Geometry check sheet. Reference: the model listing, model coordinates, mm. Face numbers are marked on the shaded views. A direction names the side the tool comes from. Round coordinates to 2 decimals unless told otherwise and drop trailing zeros. Order: outer loops, then holes, each group sorted by start corner. A loop starts at its lowest first (then second) coordinate and runs counter-clockwise, first axis right, second up. Notation, with made-up numbers: (14.25, -14.75) - (50.25, -14.75) arc R19 ccw to (50.25, -5.75) - close; hole circle Ø4 at (41, 57). An arc over 180 degrees is marked (long way). Use a Markdown table: item, result. Add a question column.
(1) Gauge pin test, flat ends, axial feed: P1, Ø1.5, axis at x = 16.5, y = 3.5, coming from the +Z side; P2, Ø1, axis at y = 3, z = 8, coming from the -X side; P3, Ø1, axis at x = 11.5, z = 8, coming from the -Y side; P4, Ø2.5, axis at x = 15.75, y = 3, coming from the -Z side. Record the tip position at first contact, or that the pin passes through.
(2) Mould release check, pull along Y, two halves, no side actions. Record for the marked faces 3, 4 and 5: released by +Y, released by -Y, zero draft, split by the parting line, or undercut.
(3) Section check C-C on z = 1.75. Give the number of separate pieces and of enclosed holes in the cut face, then the cut area to 3 significant figures.
(4) Thickness scan on line 1 along Y through (x, z) = (9.5, 4); line 2 along Z through (x, y) = (15.5, 1.5); line 3 along Y through (x, z) = (2.5, 4.75). Record the ranges inside material, lowest first. Write a range as [from, to].
(5) Access from +Z, -Z, +X, -X, +Y, -Y to the whole of each face (thin tool, end or side, straight path). Record for the marked faces 1 and 2.
(6) Section check B-B on x = 3.25. Record the boundary of the cut face in (y, z).
(7) Section check A-A on z = 7.5. Record the boundary of the cut face in (x, y).
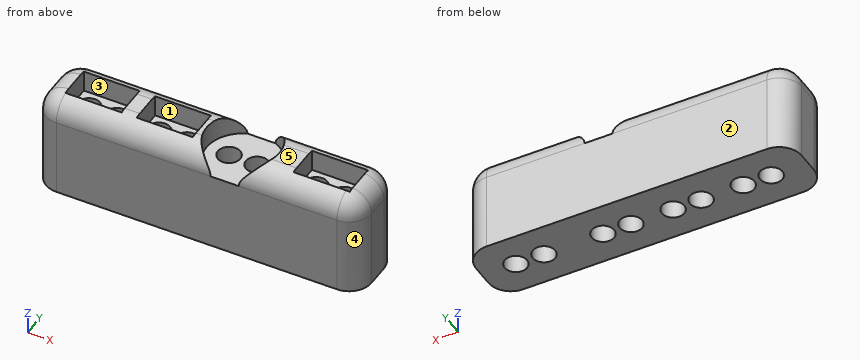
```python
from build123d import *

# Parameters (mm, degrees)
BOX001_W          = 5
BOX001_H          = 3
BOX001_DEPTH      = 10
BOX002_W          = 5
BOX002_H          = 3
BOX002_DEPTH      = 10
BOX003_W          = 5
BOX003_H          = 3
BOX003_DEPTH      = 10
CYLINDER_R        = 3.25
CYLINDER_DEPTH    = 10
CYLINDER002_R     = 1
CYLINDER002_DEPTH = 20
CYLINDER001_R     = 1
CYLINDER001_DEPTH = 20
CYLINDER004_R     = 1
CYLINDER004_DEPTH = 20
CYLINDER003_R     = 1
CYLINDER003_DEPTH = 20
CYLINDER006_R     = 1
CYLINDER006_DEPTH = 20
CYLINDER005_R     = 1
CYLINDER005_DEPTH = 20
CYLINDER008_R     = 1
CYLINDER008_DEPTH = 20
CYLINDER007_R     = 1
CYLINDER007_DEPTH = 20
BOX_W             = 29
BOX_H             = 6
BOX_DEPTH         = 9
FILLET_R          = 2


with BuildPart() as cube001:
    # Box001 → Box001 (new body)
    with BuildSketch(Plane(origin=(2, 1.5, 7), x_dir=(1, 0, 0), z_dir=(0, 0, 1))):
        with Locations((2.5, 1.5)):
            Rectangle(BOX001_W, BOX001_H)
    extrude(amount=BOX001_DEPTH)


with BuildPart() as cube002:
    # Box002 → Box002 (new body)
    with BuildSketch(Plane(origin=(8.35, 1.5, 7), x_dir=(1, 0, 0), z_dir=(0, 0, 1))):
        with Locations((2.5, 1.5)):
            Rectangle(BOX002_W, BOX002_H)
    extrude(amount=BOX002_DEPTH)


with BuildPart() as cube003:
    # Box003 → Box003 (new body)
    with BuildSketch(Plane(origin=(22.32, 1.5, 7), x_dir=(1, 0, 0), z_dir=(0, 0, 1))):
        with Locations((2.5, 1.5)):
            Rectangle(BOX003_W, BOX003_H)
    extrude(amount=BOX003_DEPTH)


with BuildPart() as cylinder:
    # Cylinder → Cylinder (new body)
    with BuildSketch(Plane(origin=(17, 3, 7), x_dir=(1, 0, 0), z_dir=(0, 0, 1))):
        Circle(CYLINDER_R)
    extrude(amount=CYLINDER_DEPTH)


with BuildPart() as cylinder002:
    # Cylinder002 → Cylinder002 (new body)
    with BuildSketch(Plane(origin=(5.75, 3, 0), x_dir=(1, 0, 0), z_dir=(0, 0, 1))):
        Circle(CYLINDER002_R)
    extrude(amount=CYLINDER002_DEPTH)


with BuildPart() as fusion:
    # Cylinder001 → Cylinder001 (new body)
    with BuildSketch(Plane(origin=(3.25, 3, 0), x_dir=(1, 0, 0), z_dir=(0, 0, 1))):
        Circle(CYLINDER001_R)
    extrude(amount=CYLINDER001_DEPTH)

    # Fusion: union Cylinder002
    add(cylinder002.part)


with BuildPart() as cylinder004:
    # Cylinder004 → Cylinder004 (new body)
    with BuildSketch(Plane(origin=(5.75, 3, 0), x_dir=(1, 0, 0), z_dir=(0, 0, 1))):
        Circle(CYLINDER004_R)
    extrude(amount=CYLINDER004_DEPTH)


with BuildPart() as fusion001:
    # Cylinder003 → Cylinder003 (new body)
    with BuildSketch(Plane(origin=(3.25, 3, 0), x_dir=(1, 0, 0), z_dir=(0, 0, 1))):
        Circle(CYLINDER003_R)
    extrude(amount=CYLINDER003_DEPTH)

    # Fusion001: union Cylinder004
    add(cylinder004.part)


with BuildPart() as fusion001_1:
    # Fusion001 placement: moved
    add(fusion001.part.moved(Location((6.25, 0, 0))))


with BuildPart() as cylinder006:
    # Cylinder006 → Cylinder006 (new body)
    with BuildSketch(Plane(origin=(5.75, 3, 0), x_dir=(1, 0, 0), z_dir=(0, 0, 1))):
        Circle(CYLINDER006_R)
    extrude(amount=CYLINDER006_DEPTH)


with BuildPart() as fusion002:
    # Cylinder005 → Cylinder005 (new body)
    with BuildSketch(Plane(origin=(3.25, 3, 0), x_dir=(1, 0, 0), z_dir=(0, 0, 1))):
        Circle(CYLINDER005_R)
    extrude(amount=CYLINDER005_DEPTH)

    # Fusion002: union Cylinder006
    add(cylinder006.part)


with BuildPart() as fusion002_1:
    # Fusion002 placement: moved
    add(fusion002.part.moved(Location((20.25, 0, 0))))


with BuildPart() as cylinder008:
    # Cylinder008 → Cylinder008 (new body)
    with BuildSketch(Plane(origin=(5.75, 3, 0), x_dir=(1, 0, 0), z_dir=(0, 0, 1))):
        Circle(CYLINDER008_R)
    extrude(amount=CYLINDER008_DEPTH)


with BuildPart() as fusion004:
    # Cylinder007 → Cylinder007 (new body)
    with BuildSketch(Plane(origin=(3.25, 3, 0), x_dir=(1, 0, 0), z_dir=(0, 0, 1))):
        Circle(CYLINDER007_R)
    extrude(amount=CYLINDER007_DEPTH)

    # Fusion003: union Cylinder008
    add(cylinder008.part)


with BuildPart() as fusion004_1:
    # Fusion003 placement: moved
    add(fusion004.part.moved(Location((12.5, 0, 0))))

    # Fusion004: union Cube001, Cube002, Cube003, Cylinder, Fusion, Fusion001, Fusion002
    add(cube001.part)
    add(cube002.part)
    add(cube003.part)
    add(cylinder.part)
    add(fusion.part)
    add(fusion001_1.part)
    add(fusion002_1.part)


with BuildPart() as standoff:
    # Box → Box (new body)
    with BuildSketch(Plane.XY):
        with Locations((14.5, 3)):
            Rectangle(BOX_W, BOX_H)
    extrude(amount=BOX_DEPTH)

    # Fillet
    fillet_edges = [standoff.edges().sort_by_distance(p)[0] for p in [
        (0, 0, 4.5),
        (0, 3, 9),
        (0, 6, 4.5),
        (29, 0, 4.5),
        (29, 3, 9),
        (29, 6, 4.5),
        (14.5, 0, 9),
        (14.5, 6, 9),
    ]]
    fillet(fillet_edges, radius=FILLET_R)

    # Cut: cut Fusion004
    add(fusion004_1.part, mode=Mode.SUBTRACT)


solid = standoff.part
```
Check sheet entries:
| question | item | result |
|---|---|---|
| 1 | P1 | stops at z = 7 |
| 1 | P2 | stops at x = 0.06 |
| 1 | P3 | stops at y = 0.06 |
| 1 | P4 | stops at z = 0 |
| 2 | face 3 | undercut |
| 2 | face 4 | released by -Y |
| 2 | face 5 | zero draft |
| 3 | separate pieces | 1 |
| 3 | enclosed holes | 8 |
| 3 | area | 145 mm2 |
| 4 | line 1 | y = [0, 2], [4, 6] |
| 4 | line 2 | z = [0, 7] |
| 4 | line 3 | y = [0, 2.34], [3.66, 6] |
| 5 | face 1 | +Z |
| 5 | face 2 | +Z, -Z, +X, -X, +Y |
| 6 | outline | (0, 0) - (2, 0) - (2, 7) - (1.5, 7) - (1.5, 8.94) arc R2 ccw to (0, 7) - close; (4, 0) - (6, 0) - (6, 7) arc R2 ccw to (4.5, 8.94) - (4.5, 7) - (4, 7) - close |
| 7 | outline | (0.06, 2) arc R1.94 ccw to (2, 0.06) - (15.61, 0.06) arc R3.25 cw to (15.61, 5.94) - (2, 5.94) arc R1.94 ccw to (0.06, 4) - close; (18.39, 0.06) - (27, 0.06) arc R1.94 ccw to (28.94, 2) - (28.94, 4) arc R1.94 ccw to (27, 5.94) - (18.39, 5.94) arc R3.25 cw to start; hole (2, 1.5) - (7, 1.5) - (7, 4.5) - (2, 4.5) - close; hole (8.35, 1.5) - (13.35, 1.5) - (13.35, 4.5) - (8.35, 4.5) - close; hole (22.32, 1.5) - (27.32, 1.5) - (27.32, 4.5) - (22.32, 4.5) - close |
